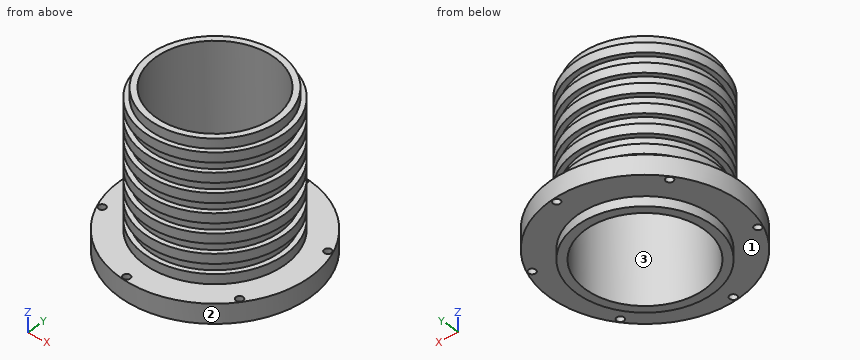
```python
from build123d import *

# Parameters (mm, degrees)
SKETCH1_R           = 28
BOSS_EXTRUDE1_DEPTH = 4
SKETCH2_R           = 39.25
BOSS_EXTRUDE2_DEPTH = 8
SKETCH4_R           = 27
BOSS_EXTRUDE3_DEPTH = 56
SKETCH5_R           = 24.5
CUT_EXTRUDE2_DEPTH  = 88.778841414
SKETCH6_R           = 29
BOSS_EXTRUDE4_DEPTH = 4
LPATTERN1_COUNT     = 7
LPATTERN1_PITCH     = 8
SKETCH8_R           = 1.5
CUT_EXTRUDE3_DEPTH  = 79.848747612
CIRPATTERN1_COUNT   = 6
SKETCH9_R           = 24.5
CUT_EXTRUDE4_DEPTH  = 85.71791428


with BuildPart() as part:
    # Sketch1 → Boss-Extrude1 (new body)
    with BuildSketch(Plane.XY):
        Circle(SKETCH1_R)
    extrude(amount=BOSS_EXTRUDE1_DEPTH)

    # Sketch2 → Boss-Extrude2 (add)
    with BuildSketch(Plane.XY.offset(4)):
        Circle(SKETCH2_R)
    extrude(amount=BOSS_EXTRUDE2_DEPTH)

    # Sketch4 → Boss-Extrude3 (add)
    with BuildSketch(Plane.XY.offset(12)):
        Circle(SKETCH4_R)
    extrude(amount=BOSS_EXTRUDE3_DEPTH)

    # Sketch5 → Cut-Extrude2 (cut, through all)
    with BuildSketch(Plane.XY.offset(68)):
        Circle(SKETCH5_R)
    extrude(amount=-CUT_EXTRUDE2_DEPTH, mode=Mode.SUBTRACT)

    # Sketch6 → Boss-Extrude4 (add)
    with BuildSketch(Plane.XY.offset(12)):
        Circle(SKETCH6_R)
    boss_extrude4 = extrude(amount=BOSS_EXTRUDE4_DEPTH)

    # LPattern1: Boss-Extrude4 ×7
    with Locations(*[(0, 0, i * LPATTERN1_PITCH) for i in range(1, LPATTERN1_COUNT)]):
        add(boss_extrude4)

    # Sketch8 → Cut-Extrude3 (cut, through all)
    with BuildSketch(Plane.XY.offset(12)):
        with Locations((4.985240287, 37.167154576)):
            Circle(SKETCH8_R)
    cut_extrude3 = extrude(amount=-CUT_EXTRUDE3_DEPTH, mode=Mode.SUBTRACT)

    # CirPattern1: Cut-Extrude3 ×6 about axis
    cirpattern1_axis = Axis((0, 0, 0), (0, 0, 1))
    for i in range(1, CIRPATTERN1_COUNT):
        add(cut_extrude3.rotate(cirpattern1_axis, i * 360 / CIRPATTERN1_COUNT), mode=Mode.SUBTRACT)

    # Sketch9 → Cut-Extrude4 (cut, through all)
    with BuildSketch(Plane.XY.offset(64)):
        Circle(SKETCH9_R)
    extrude(amount=-CUT_EXTRUDE4_DEPTH, mode=Mode.SUBTRACT)


solid = part.part
```
The model under review builds one solid part; all positions refer to its coordinate system, in mm. Face numbers are marked on the shaded views. Coordinates: 2 decimals unless noted, no trailing zeros. Order: outer loops, then holes, each group sorted by start corner. A loop starts at its lowest first (then second) coordinate and runs counter-clockwise, first axis right, second up. Notation, with made-up numbers: (-27, -14) -> (-14, -14) arc R17 ccw to (-14, 12) -> close; hole circle Ø1 at (39.25, 46). An arc over 180 degrees is marked (long way). Answer in a Markdown table with one row per item. Add a question column.
Item 1: Mouldability with a two-part tool opening along Y and no side actions: class the marked faces 1, 2 and 3 as +Y half, -Y half, draft (parallel to the pull), parting line (faces both ways), or undercut.
Item 2: To check wall thickness, follow probe 1 along Z at (x, y) = (-13.5, -36); probe 2 along X at (y, z) = (14, 17.5); probe 3 along X at (y, z) = (5.5, 11). State the ranges of each line that lie inside material, in increasing order.
Item 3: Clearance check with flat-ended pins moving along their axes: pin 1 (1 mm diameter, centred on x = 11.5, z = 23.5, fed in from -Y); pin 2 (1.5 mm diameter, centred on x = -1.5, z = 8.5, fed in from +Y); pin 3 (6 mm diameter, centred on x = -1.5, z = 59.5, fed in from +Y). State where each tip first meets the part, or that it passes through.
Item 4: We need section B-B on y = 31. Write out the cut boundary in (x, z).
Item 5: We need section A-A on z = 25.5. Write out the cut boundary in (x, y), plus the area to 3 significant figures.
Final values:
| question | item | result |
|---|---|---|
| 1 | face 1 | draft |
| 1 | face 2 | parting line |
| 1 | face 3 | undercut |
| 2 | probe 1 | z = 4 to 12 |
| 2 | probe 2 | x = -23.09 to -20.11, 20.11 to 23.09 |
| 2 | probe 3 | x = -38.86 to -23.87, 23.87 to 38.86 |
| 3 | pin 1 | stops at y = -26.83 |
| 3 | pin 2 | stops at y = 39.24 |
| 3 | pin 3 | stops at y = 29 |
| 4 | outline | (-24.07, 4) -> (24.07, 4) -> (24.07, 12) -> (-24.07, 12) -> close |
| 5 | outline | circle Ø54 at (0, 0); hole circle Ø49 at (0, 0) |
| 5 | area | 404 mm2 |
